Verification items for the finished model (mm, model axes). Round coordinates to 2 decimals unless told otherwise and drop trailing zeros. Write each loop counter-clockwise with the first axis right and the second up, starting at its lowest first coordinate (ties: lowest second). Pieces come first, ordered by that corner, then holes.
from build123d import *

# Parameters (mm, degrees)
SKETCH3_R                = 1.5
BOSS_EXTRUDE1_DEPTH      = 6.35
M3_CLEARANCE_HOLE1_D     = 3.2
M3_CLEARANCE_HOLE1_DEPTH = 7.5
M3_CLEARANCE_HOLE1_TIP   = 0.96137699


with BuildPart() as part:
    # Sketch3 → Boss-Extrude1 (new body)
    with BuildSketch(Plane.XY):
        with BuildLine():
            Line((61.771243445, -15), (-61.771243445, -15))
            ThreePointArc((-61.771243445, -15), (-95, 0), (-61.771243445, 15))
            Line((-61.771243445, 15), (61.771243445, 15))
            ThreePointArc((61.771243445, 15), (95, 0), (61.771243445, -15))
        make_face()
        with Locations((-20, 0)):
            Circle(SKETCH3_R, mode=Mode.SUBTRACT)
        with Locations((20, 0)):
            Circle(SKETCH3_R, mode=Mode.SUBTRACT)
    extrude(amount=BOSS_EXTRUDE1_DEPTH)

    # M3 Clearance Hole1
    with Locations(Plane.XY.offset(6.35)):
        with Locations((75, 0), (-75, 0), (-81.717514421, -6.717514421), (-69.343145751, -5.656854249), (-68.282485579, 6.717514421), (-80.656854249, 5.656854249), (0, 0), (81.717514421, 6.717514421), (69.343145751, 5.656854249), (68.282485579, -6.717514421), (80.656854249, -5.656854249)):
            Hole(M3_CLEARANCE_HOLE1_D / 2, depth=M3_CLEARANCE_HOLE1_DEPTH)
            with Locations((0, 0, -(M3_CLEARANCE_HOLE1_DEPTH + M3_CLEARANCE_HOLE1_TIP / 2))):  # 118° drill point
                Cone(0, M3_CLEARANCE_HOLE1_D / 2, M3_CLEARANCE_HOLE1_TIP, mode=Mode.SUBTRACT)


solid = part.part
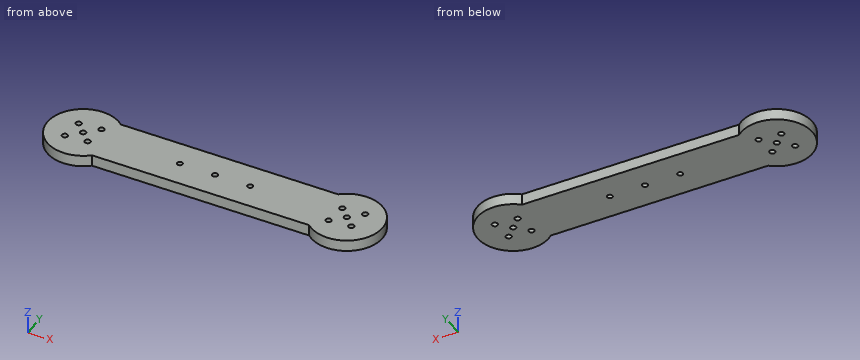
Q1. Sectioned sample at A-A (x = -75). Enter the section's corners in (y, z), plus the area to 3 significant figures.
Recorded:
outline: (-20, 0) - (-1.6, 0) - (-1.6, 6.35) - (-20, 6.35) - close; (1.6, 0) - (20, 0) - (20, 6.35) - (1.6, 6.35) - close
area: 234 mm2
Q2. Depth check by flat-ended pin: P1, Ø2, axis at x = 37.5, z = 5.5, coming from the -Y side; P2, Ø3, axis at x = 10.5, z = 3, coming from the +Y side; P3, Ø1, axis at y = 1.5, z = 4.5, coming from the -X side (3 decimals). Enter the tip coordinate at first touch or a pass-through.
Recorded:
P1: stops at y = -15
P2: stops at y = 15
P3: stops at x = -94.975
Q3. Sectioned sample at B-B (z = 1.5). Give the number of separate pieces and of enclosed holes in the cut face, plus the area to 3 significant figures.
Recorded:
separate pieces: 1
enclosed holes: 13
area: 5,840 mm2
Q4. Sectioned sample at D-D (x = -45). Enter the section's corners in (y, z).
Recorded:
outline: (-15, 0) - (15, 0) - (15, 6.35) - (-15, 6.35) - close
Q5. Material ranges on line 1 along X through (y, z) = (-6, 6); line 2 along Y through (x, z) = (75, 4.5); line 3 along X through (y, z) = (-1, 2.75), recorded low to high.
Recorded:
line 1: x = -94.08 to -83.15, -80.29 to -70.91, -67.78 to 66.85, 69.71 to 79.09, 82.22 to 94.08
line 2: y = -20 to -1.6, 1.6 to 20
line 3: x = -94.97 to -76.25, -73.75 to -21.12, -18.88 to -1.25, 1.25 to 18.88, 21.12 to 73.75, 76.25 to 94.97
Q6. Sectioned sample at C-C (x = 0). Enter the section's corners in (y, z).
Recorded:
outline: (-15, 0) - (-1.6, 0) - (-1.6, 6.35) - (-15, 6.35) - close; (1.6, 0) - (15, 0) - (15, 6.35) - (1.6, 6.35) - close
